Read the model definition and answer for the solid it produces. Units are mm, in the model's axes. A direction names the side the tool comes from. Coordinates: 2 decimals unless noted, no trailing zeros. Loops run counter-clockwise (first coordinate to the right, second up) from the corner with the lowest first, then second, coordinate; pieces in that order, holes last. Notation, with made-up numbers: (55, 15.25) - (111, 15.25) arc R24 cw to (111, 27.25) - close; hole circle Ø8 at (1, 25.25). An arc over 180 degrees is marked (long way). Use one line per item in the form item = value.
from build123d import *

# Parameters (mm, degrees)
SKETCH_1_R               = 17
SKETCH_1_R_2             = 7
SKETCH_1_R_3             = 1.6
EXTRUDE_1_DEPTH          = 2
EXTRUDE_START            = 40.5
SKETCH_2_R               = 17
SKETCH_2_R_2             = 15
EXTRUDE_2_DEPTH          = 40.5
EXTRUDE_3_REACH          = 82.114
EXTRUDE_3_END_RADIUS     = 17
SKETCH_5_W               = 4
SKETCH_5_H               = 12
EXTRUDE_4_DEPTH          = 2
CUT_EXTRUDE_1_REACH      = 83.143
SKETCH_6_W               = 16
SKETCH_6_H               = 8
SKETCH_7_W               = 12
SKETCH_7_H               = 2
EXTRUDE_5_DEPTH          = 2
MIRROR_2_COPY_1_SKETCH_W = 12
MIRROR_2_COPY_1_SKETCH_H = 2
MIRROR_2_COPY_1_DEPTH    = 2
MIRROR_2_COPY_2_SKETCH_W = 12
MIRROR_2_COPY_2_SKETCH_H = 2
MIRROR_2_COPY_2_DEPTH    = 2
FILLET_1_R               = 10


with BuildPart() as part:
    # 草图1 → 凸台-拉伸1 (new body)
    with BuildSketch(Plane(origin=(0, 0, 0), x_dir=(1, 0, 0), z_dir=(0, 1, 0))):
        with Locations(Location((0, 0, 0), (0, 0, 270))):
            Circle(SKETCH_1_R)
        with Locations(Location((0, 0, 0), (0, 0, 270))):
            Circle(SKETCH_1_R_2, mode=Mode.SUBTRACT)
        with Locations(Location((9.17629535, -2.458780928, 0), (0, 0, 270))):
            Circle(SKETCH_1_R_3, mode=Mode.SUBTRACT)
        with Locations(Location((-6.717514421, -6.717514421, 0), (0, 0, 270))):
            Circle(SKETCH_1_R_3, mode=Mode.SUBTRACT)
        with Locations(Location((-2.458780928, 9.17629535, 0), (0, 0, 270))):
            Circle(SKETCH_1_R_3, mode=Mode.SUBTRACT)
    extrude(amount=-EXTRUDE_1_DEPTH)

    # 草图2 → 凸台-拉伸2 (add)
    with BuildSketch(Plane(origin=(0, 0, 0), x_dir=(1, 0, 0), z_dir=(0, 1, 0)).offset(EXTRUDE_START)):
        with Locations(Location((0, 0, 0), (0, 0, 270))):
            Circle(SKETCH_2_R)
        with Locations(Location((0, 0, 0), (0, 0, 270))):
            Circle(SKETCH_2_R_2, mode=Mode.SUBTRACT)
    extrude(amount=-EXTRUDE_2_DEPTH)

    # 凸台-拉伸3: up to this cylinder (the profile starts outside it)
    extrude_3_end = Plane(origin=(0, 40.276393, 0), z_dir=(0, 1, 0)) * Cylinder(EXTRUDE_3_END_RADIUS, 199.228, mode=Mode.PRIVATE)
    # 草图4 → 凸台-拉伸3 (add, up to the surface)
    with BuildSketch(Plane(origin=(50, 0, 0), x_dir=(0, 0, -1), z_dir=(1, 0, 0)), mode=Mode.PRIVATE) as extrude_3_sk1:
        Polygon((-10, 40.5), (-8, 40.5), (-8, 32.5), (8, 32.5), (8, 40.5), (10, 40.5), (10, 30.5), (-10, 30.5), align=None)
    extrude_3_tool1 = extrude(extrude_3_sk1.sketch, amount=-EXTRUDE_3_REACH, mode=Mode.PRIVATE) - extrude_3_end
    extrude_3 = extrude_3_tool1.solids().sort_by_distance((50, 40.276393, 9))[0]
    add(extrude_3)

    # 草图5 → 凸台-拉伸4 (add)
    with BuildSketch(Plane(origin=(50, 0, 0), x_dir=(0, 0, -1), z_dir=(1, 0, 0))):
        with Locations((-10, 36.5)):
            Rectangle(SKETCH_5_W, SKETCH_5_H)
        with Locations((10, 36.5)):
            Rectangle(SKETCH_5_W, SKETCH_5_H)
    extrude_4 = extrude(amount=EXTRUDE_4_DEPTH)

    # 草图6 → 切除-拉伸1 (cut, up to next)
    with BuildSketch(Plane(origin=(50, 0, 0), x_dir=(0, 0, -1), z_dir=(1, 0, 0)), mode=Mode.PRIVATE) as cut_extrude_1_sk1:
        with Locations((0, 36.5)):
            Rectangle(SKETCH_6_W, SKETCH_6_H)
    cut_extrude_1_tool1 = extrude(cut_extrude_1_sk1.sketch, amount=-CUT_EXTRUDE_1_REACH, mode=Mode.PRIVATE) & part.part
    cut_extrude_1 = cut_extrude_1_tool1.solids().sort_by_distance((50, 36.5, 0))[0]
    add(cut_extrude_1, mode=Mode.SUBTRACT)

    # 草图7 → 凸台-拉伸5 (add)
    with BuildSketch(Plane(origin=(0, 40.5, 0), x_dir=(1, 0, 0), z_dir=(0, 1, 0))):
        with Locations((31.873863542, -9)):
            Rectangle(SKETCH_7_W, SKETCH_7_H)
    extrude_5 = extrude(amount=EXTRUDE_5_DEPTH)

    # 镜向1: 凸台-拉伸5 across plane
    add(extrude_5.mirror(Plane.XY))

    # 镜向2: 凸台-拉伸3, 凸台-拉伸4, 切除-拉伸1 across plane
    add(extrude_3.mirror(Plane(origin=(0, 0, 0), x_dir=(0, 0, 1), z_dir=(1, 0, 0))))
    add(extrude_4.mirror(Plane(origin=(0, 0, 0), x_dir=(0, 0, 1), z_dir=(1, 0, 0))))
    add(cut_extrude_1.mirror(Plane(origin=(0, 0, 0), x_dir=(0, 0, 1), z_dir=(1, 0, 0))), mode=Mode.SUBTRACT)

    # 镜向2 copy 1 sketch → 镜向2 copy 1 (add)
    with BuildSketch(Plane(origin=(0, 40.5, 0), x_dir=(-1, 0, 0), z_dir=(0, 1, 0))):
        with Locations((31.873863542, -9)):
            Rectangle(MIRROR_2_COPY_1_SKETCH_W, MIRROR_2_COPY_1_SKETCH_H)
    extrude(amount=MIRROR_2_COPY_1_DEPTH)

    # 镜向2 copy 2 sketch → 镜向2 copy 2 (add)
    with BuildSketch(Plane(origin=(0, 40.5, 0), x_dir=(-1, 0, 0), z_dir=(0, 1, 0))):
        with Locations((31.873863542, 9)):
            Rectangle(MIRROR_2_COPY_2_SKETCH_W, MIRROR_2_COPY_2_SKETCH_H)
    extrude(amount=MIRROR_2_COPY_2_DEPTH)

    # 圆角1
    fillet_1_edges = [part.edges().sort_by_distance(p)[0] for p in [
        (-13.747727085, 35.5, 10),
        (-13.747727085, 35.5, -10),
        (-17, 30.5, 0),
        (13.747727085, 35.5, 10),
        (13.747727085, 35.5, -10),
        (17, 30.5, 0),
    ]]
    fillet(fillet_1_edges, radius=FILLET_1_R)


solid = part.part
Item 1: Find the intervals of material crossed by L1, parallel to X at y = 10, z = 0; L2, parallel to X at y = 25.5, z = -9; L3, parallel to Y at x = 35, z = 9, in increasing order.
Results below:
L1 = -17 to -15, 15 to 17
L2 = -15.98 to -12, 12 to 15.98
L3 = 30.5 to 42.5
Item 2: Each of these flat-tipped pins is pushed along its axis until it touches: P1, Ø8, axis at x = 37, y = 33.5, coming from the -Z side; P2, Ø9, axis at x = 6.5, z = -3.5, coming from the +Y side; P3, Ø1, axis at x = 51.5, y = 36.5, coming from the +Z side. Where does it stop, or does it pass through?
Results below:
P1 = -10
P2 = 0
P3 = 12
Item 3: Which of the six approach directions +Z, -Z, +X, -X, +Y, -Y give full straight-line access (tool end or side, diameter ignored) to faces 4 (the flat face through (-32, 32.5, 0)), 5 (the flat face through (-25.874, 41, -9)), 6 (the flat face through (50, 38, -11)), 7 (the cylindrical face through (-15, 15, 8)), 8 (the flat face through (-34, 35, 10))?
Results below:
face_4 = +X, -X, +Y
face_5 = +Z, -Z, +Y
face_6 = -Z, +Y
face_7 = -Y
face_8 = +Z, +Y, -Y
Item 4: The part is cut by section C-C on y = 24.5. Give the vertices of the cut face in (x, z).
Results below:
outline = (-14.18, -10.82) arc R10 cw to (-11.42, -12.59) arc R17 ccw to (11.42, -12.59) arc R10 cw to (14.18, -10.82) arc R17.83 ccw to (14.18, 10.82) arc R10 cw to (11.42, 12.59) arc R17 ccw to (-11.42, 12.59) arc R10 cw to (-14.18, 10.82) arc R17.83 ccw to start; hole circle Ø30 at (0, 0)
Item 5: The part is cut by section A-A on y = 34.5. Give the vertices of the cut face in (x, z).
Results below:
outline = (-52, -12) - (-50, -12) - (-50, -10) - (-18.14, -10) arc R10 cw to (-11.42, -12.59) arc R17 ccw to (11.42, -12.59) arc R10 cw to (18.14, -10) - (50, -10) - (50, -12) - (52, -12) - (52, -8) - (12.69, -8) arc R15 cw to (-12.69, -8) - (-52, -8) - close; (-52, 8) - (-12.69, 8) arc R15 cw to (12.69, 8) - (52, 8) - (52, 12) - (50, 12) - (50, 10) - (18.14, 10) arc R10 cw to (11.42, 12.59) arc R17 ccw to (-11.42, 12.59) arc R10 cw to (-18.14, 10) - (-50, 10) - (-50, 12) - (-52, 12) - close
Item 6: For a pull along X with two mould halves and no side action, classify faces 1 (the flat face through (-52, 37, 10)), 2 (the flat face through (51, 36, 12)), 3 (the flat face through (25.874, 41, 9)) as +X half, -X half, draft (parallel to the pull), parting line (faces both ways), or undercut.
Results below:
face_1 = -X half
face_2 = draft
face_3 = undercut
Item 7: The part is cut by section B-B on y = 19. Give the vertices of the cut face in (x, z), plus the area to 3 significant figures.
Results below:
outline = circle Ø34 at (0, 0); hole circle Ø30 at (0, 0)
area = 201 mm²
